Could you check a few things on this drawing? It's one solid part, dimensions in mm from its lowest x, y, z. A direction names the side the tool comes from. Round coordinates to 2 decimals unless told otherwise and drop trailing zeros. Loops run counter-clockwise (first coordinate to the right, second up) from the corner with the lowest first, then second, coordinate; pieces in that order, holes last. Notation, with made-up numbers: M 85.25,77 L 127.25,77 A14 ccw 127.25,85 Z; hole C 63,20.25 d7. An arc over 180 degrees is marked long. Write each question's results on one line, items separated by ' | '. Start each with the question number.
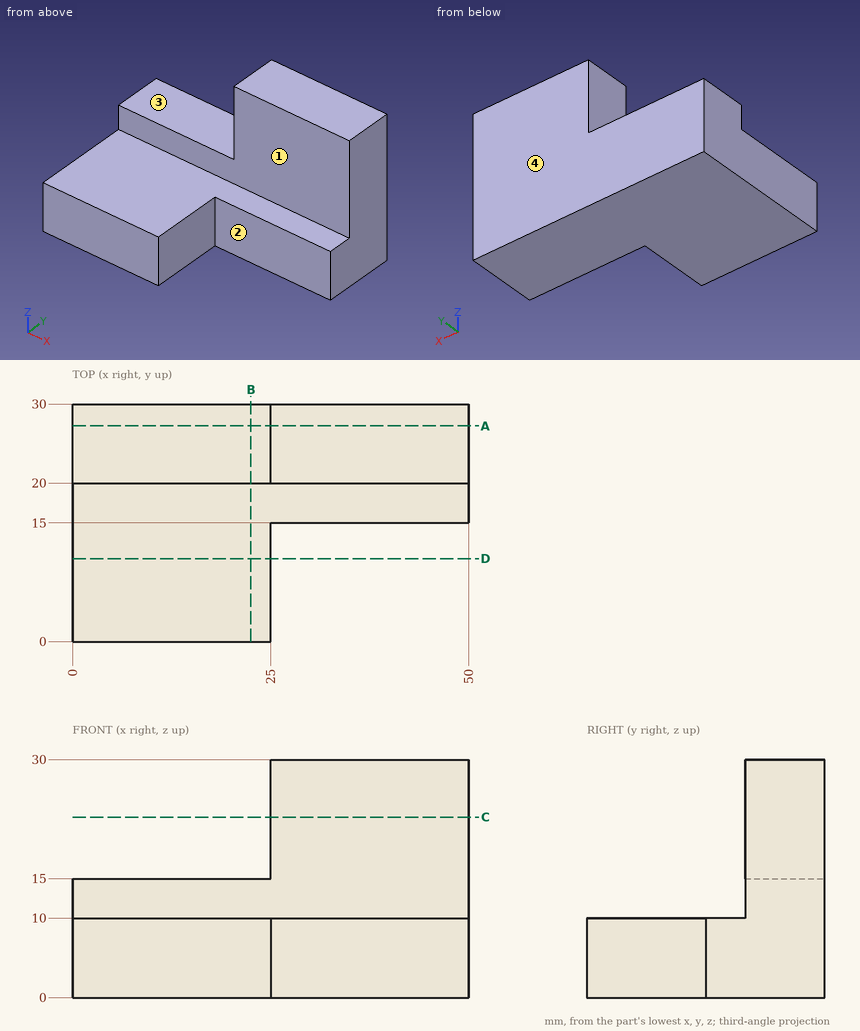
1. Which directions (+Z, -Z, +X, -X, +Y, -Y) give clear straight access to the entire face, cutting with the end or side of a thin tool? Please do the marked faces 1, 2, 3 and 4.
2. I want a section at A-A on y = 27.25. List the corners of the cut face in (x, z) for me, plus the area to 4 significant figures.
3. I need wall thicknesses on line 1 along X through (y, z) = (26.25, 18.75); line 2 along Y through (x, z) = (34.5, 8.25); line 3 along Z through (x, y) = (17.5, 6). Which ranges of each line are inside material? Lowest first, please.
4. I want a section at C-C on z = 22.75. List the corners of the cut face in (x, y) for me, plus the area to 3 significant figures.
5. I want a section at B-B on x = 22.5. List the corners of the cut face in (y, z) for me, plus the area to 3 significant figures.
6. I want a section at D-D on y = 10.5. List the corners of the cut face in (x, z) for me.
7. For pin 1 (8 mm diameter, centred on y = 26, z = 22, fed in from -X); pin 2 (3 mm diameter, centred on x = 12, z = 17.5, fed in from +Y); pin 3 (8 mm diameter, centred on x = 12.5, y = 23.5, fed in from +Z); pin 4 (6 mm diameter, centred on x = 18, y = 5, fed in from +Z), each with a flat end and sliding along its axis, tell me the tip position at first contact or that it passes through.
Outcome:
1) face 1: +Z, +X, -X, -Y | face 2: +Z, -Z, +X, -Y | face 3: +Z, -X, +Y, -Y | face 4: +Z, -Z, +X, -X, +Y
2) outline: M 0,0 L 50,0 L 50,30 L 25,30 L 25,15 L 0,15 Z | area: 1,125 mm2
3) line 1: 25 to 50 | line 2: 15 to 30 | line 3: 0 to 10
4) outline: M 25,20 L 50,20 L 50,30 L 25,30 Z | area: 250 mm2
5) outline: M 0,0 L 30,0 L 30,15 L 20,15 L 20,10 L 0,10 Z | area: 350 mm2
6) outline: M 0,0 L 25,0 L 25,10 L 0,10 Z
7) pin 1: x = 25 | pin 2: through | pin 3: z = 15 | pin 4: z = 10
